```python
from build123d import *

# Parameters (mm, degrees)
EXTRUDE_1_DEPTH = 1.2
SKETCH_2_R      = 4.5
EXTRUDE_2_DEPTH = 6


with BuildPart() as part:
    # 草图1 → 凸台-拉伸1 (new body)
    with BuildSketch(Plane(origin=(0, 0, 0), x_dir=(1, 0, 0), z_dir=(0, 1, 0))):
        with BuildLine():
            Line((-12, 0), (-9.741657387, 0))
            ThreePointArc((-9.741657387, 0), (-6, -2), (-2.258342613, 0))
            Line((-2.258342613, 0), (0, 0))
            Line((0, 0), (0, 5))
            Line((0, 5), (-2.258342613, 5))
            ThreePointArc((-2.258342613, 5), (-6, 7), (-9.741657387, 5))
            Line((-9.741657387, 5), (-12, 5))
            Line((-12, 5), (-12, 0))
        make_face()
    extrude(amount=EXTRUDE_1_DEPTH)

    # 草图2 → 凸台-拉伸2 (add)
    with BuildSketch(Plane(origin=(0, 1.2, 0), x_dir=(1, 0, 0), z_dir=(0, 1, 0))):
        with Locations(Location((-6, 2.5, 0), (0, 0, 146.251011404))):
            Circle(SKETCH_2_R)
    extrude(amount=EXTRUDE_2_DEPTH)


solid = part.part
```
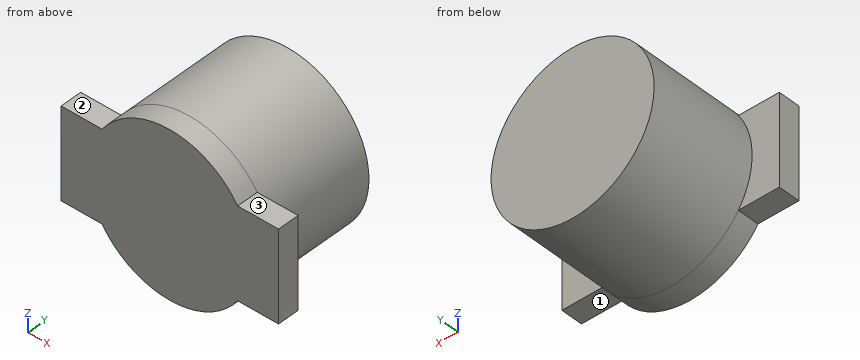
Geometry check sheet. Reference: the model listing, model coordinates, mm. Face numbers are marked on the shaded views. A direction names the side the tool comes from. Coordinates: 2 decimals unless noted, no trailing zeros. Order: outer loops, then holes, each group sorted by start corner. A loop starts at its lowest first (then second) coordinate and runs counter-clockwise, first axis right, second up. Notation, with made-up numbers: (4, 4.5) - (8, 4.5) arc R21 cw to (8, 8.5) - close; hole circle Ø3 at (-2.75, 30). An arc over 180 degrees is marked (long way). Use one line per item in the form item = value.
1. Section check B-B (x = -0.75). Record the boundary of the cut face in (y, z), then the cut area to 3 significant figures.
Here are the results:
outline = (0, -5) - (1.2, -5) - (1.2, 0) - (0, 0) - close
area = 6.00 mm²
2. Section check A-A (z = -2.5). Record the boundary of the cut face in (x, y), then the cut area to 3 significant figures.
Here are the results:
outline = (-12, 0) - (0, 0) - (0, 1.2) - (-1.5, 1.2) - (-1.5, 7.2) - (-10.5, 7.2) - (-10.5, 1.2) - (-12, 1.2) - close
area = 68.4 mm²
3. Section check C-C (y = 2.5). Record the boundary of the cut face in (x, z).
Here are the results:
outline = circle Ø9 at (-6, -2.5)
4. Scan lines: line 1 (Y direction, x = -10.5, z = -1.25); line 2 (X direction, y = 2.5, z = -5); line 3 (X direction, y = 3.5, z = -2.25). Record each from-to range of solid material in increasing order.
Here are the results:
line_1 = 0 to 1.2
line_2 = -9.74 to -2.26
line_3 = -10.49 to -1.51
5. Gauge pin test, flat ends, axial feed: pin 1 (1 mm diameter, centred on x = -0.5, y = 0.5, fed in from +Z); pin 2 (0.7 mm diameter, centred on x = -0.5, z = -2, fed in from +Y); pin 3 (1.5 mm diameter, centred on x = -3, y = 3.5, fed in from -Z). Record the tip position at first contact, or that the pin passes through.
Here are the results:
pin_1 = 0
pin_2 = 1.2
pin_3 = -6.4
6. Section check D-D (z = -1). Record the boundary of the cut face in (x, y), then the cut area to 3 significant figures.
Here are the results:
outline = (-12, 0) - (0, 0) - (0, 1.2) - (-1.76, 1.2) - (-1.76, 7.2) - (-10.24, 7.2) - (-10.24, 1.2) - (-12, 1.2) - close
area = 65.3 mm²
7. Access from +Z, -Z, +X, -X, +Y, -Y to the whole of each face (thin tool, end or side, straight path). Record for the marked faces 1, 2 and 3.
Here are the results:
face_1 = -Z, +X, +Y, -Y
face_2 = +Z, -X, +Y, -Y
face_3 = +Z, +X, +Y, -Y
